```python
from build123d import *

# Parameters (mm, degrees)
F0_W     = 314.96
F0_H     = 101.6
F0_W_2   = 39.116
F0_H_2   = 71.12
F0_R     = 4.7625
F1_DEPTH = 5.08
F2_D     = 3.302
F3_D     = 6.35


with BuildPart() as f1:
    # F0 (on Top) → F1 (new body)
    with BuildSketch(Plane.XY):
        with Locations((25.4, -8.1075665182)):
            Rectangle(F0_W, F0_H)
        with Locations((47.752, -8.1075665182)):
            Rectangle(F0_W_2, F0_H_2, mode=Mode.SUBTRACT)
        with Locations((99.568, -8.1075665182)):
            Rectangle(F0_W_2, F0_H_2, mode=Mode.SUBTRACT)
        with Locations((151.13, -8.1075665182)):
            Circle(F0_R, mode=Mode.SUBTRACT)
    extrude(amount=F1_DEPTH)

    # F2 (through all)
    with Locations(Plane(origin=(0, 0, 0), x_dir=(1, 0, 0), z_dir=(0, 0, -1))):
        with Locations((-120.65, -33.8024334818), (-22.86, -33.8024334818), (73.66, -33.8024334818), (171.45, -33.8024334818), (171.45, 50.0175665182), (73.66, 50.0175665182), (-22.86, 50.0175665182), (-120.65, 50.0175665182)):
            Hole(F2_D / 2)

    # F3 (through all)
    with Locations(Plane(origin=(0, 0, 0), x_dir=(1, 0, 0), z_dir=(0, 0, -1))):
        with Locations((15.494, -10.9424334818), (15.494, 27.1575665182)):
            Hole(F3_D / 2)


solid = f1.part
```
Model file for the job. Use its own axes, mm. A direction names the side the tool comes from. Give positions to 0.01 mm unless a question says otherwise; leave off trailing zeros. Write each loop counter-clockwise with the first axis right and the second up, starting at its lowest first coordinate (ties: lowest second). Pieces come first, ordered by that corner, then holes. Notation, with made-up numbers: M 78,-37 L 88,-37 A10 ccw 88,-29 Z; hole C -25,10 d10. An arc over 180 degrees is marked long. Use a Markdown table: item, result.
1) Tool access for faces 4 (the flat face through (23, -58.908, 3)), 5 (the flat face through (99, 27.452, 3)): list every direction of +Z, -Z, +X, -X, +Y, -Y with a clear straight run to the whole face (end or side of a thin tool).
Responses:
| item | result |
|---|---|
| face 4 | +Z, -Z, +X, -X, -Y |
| face 5 | +Z, -Z |
2) Drill centre lines: line 1 (X direction, y = 23, z = 0.7); line 2 (Y direction, x = -120.65, z = 2.2); line 3 (X direction, y = -8, z = 4.7). Where is each one in solid material? Low to high. Write a range as from..to.
Responses:
| item | result |
|---|---|
| line 1 | x = -132.08..28.19, 67.31..80.01, 119.13..182.88 |
| line 2 | y = -58.91..-51.67, -48.37..32.15, 35.45..42.69 |
| line 3 | x = -132.08..28.19, 67.31..80.01, 119.13..146.37, 155.89..182.88 |
3) Cut at D-D (x = 151.13). List the corners of the cut face in (y, z).
Responses:
| item | result |
|---|---|
| outline | M -58.91,0 L -12.87,0 L -12.87,5.08 L -58.91,5.08 Z; M -3.35,0 L 42.69,0 L 42.69,5.08 L -3.35,5.08 Z |
4) Cut at A-A (x = 53). List the corners of the cut face in (y, z).
Responses:
| item | result |
|---|---|
| outline | M -58.91,0 L -43.67,0 L -43.67,5.08 L -58.91,5.08 Z; M 27.45,0 L 42.69,0 L 42.69,5.08 L 27.45,5.08 Z |
5) Cut at B-B (y = -18). List the corners of the cut face in (x, z).
Responses:
| item | result |
|---|---|
| outline | M -132.08,0 L 28.19,0 L 28.19,5.08 L -132.08,5.08 Z; M 67.31,0 L 80.01,0 L 80.01,5.08 L 67.31,5.08 Z; M 119.13,0 L 182.88,0 L 182.88,5.08 L 119.13,5.08 Z |
6) Pin check, flat tip, straight feed: pin 1 (12 mm diameter, centred on x = 85.5, y = 6.5, fed in from -Z). Stop position of the tip, or through.
Responses:
| item | result |
|---|---|
| pin 1 | stops at z = 0 |
7) Pull direction X, two halves, no side cores. Call faces 1 (the flat face through (182.88, -9, 3)), 2 (the flat face through (-132.08, -9, 3)), 3 (the flat face through (28.194, -9, 3)): +X half, -X half, draft (parallel to the pull), parting line (faces both ways), or undercut.
Responses:
| item | result |
|---|---|
| face 1 | +X half |
| face 2 | -X half |
| face 3 | undercut |
8) Cut at C-C (z = 1.3). Give the number of separate pieces and of enclosed holes in the cut face, and give its area (3 significant figures).
Responses:
| item | result |
|---|---|
| separate pieces | 1 |
| enclosed holes | 13 |
| area | 26,200 mm2 |
